```python
from build123d import *

# Parameters (mm, degrees)
F0_R     = 15.875
F1_DEPTH = 44.45
F2_SIZE  = 4.7625
F3_R     = 1.5875
F4_DEPTH = 17


with BuildPart() as f1:
    # F0 (on Front) → F1 (new body)
    with BuildSketch(Plane.XZ):
        Circle(F0_R)
    extrude(amount=F1_DEPTH)

    # F2
    f2_edges = [f1.edges().sort_by_distance(p)[0] for p in [
        (-15.875, -44.45, 0),
    ]]
    chamfer(f2_edges, length=F2_SIZE)

    # F3 (on face) → F4 (join)
    with BuildSketch(Plane.XZ.offset(44.45)):
        Circle(F3_R)
    extrude(amount=F4_DEPTH)


solid = f1.part
```
Model file for the job. Use its own axes, mm. A direction names the side the tool comes from. Coordinates: 2 decimals unless noted, no trailing zeros. Loops run counter-clockwise (first coordinate to the right, second up) from the corner with the lowest first, then second, coordinate; pieces in that order, holes last. Notation, with made-up numbers: (22.25, 45) - (47.25, 45) arc R21 cw to (47.25, 54) - close; hole circle Ø11 at (-4, 58). An arc over 180 degrees is marked (long way). Answer as a JSON object with one key per item and string values. Group by question number.
(1) Tool access for faces 1 (the face through (-0.34, -52.83, -1.55)), 2 (the face through (-3.441, -19.566, -15.497)): list every direction of +Z, -Z, +X, -X, +Y, -Y with a clear straight run to the whole face (end or side of a thin tool).
(2) Flat gauge pins, fed straight in: pin 1 (8 mm diameter, centred on x = 9.5, y = -34.5, fed in from -Z); pin 2 (3 mm diameter, centred on y = -20, z = 12.5, fed in from +X); pin 3 (12 mm diameter, centred on x = 10.5, y = -7, fed in from -Z). Where does each tip first touch, or does it go through?
(3) Cut at C-C (y = -35). Give the cut face in (x, z) (3 decimals), then the cut area to 3 significant figures.
(4) Cut at D-D (y = -48.5). Give the cut face in (x, z) (1 decimal).
(5) Probe line 1 along Y through (x, z) = (-6, -3.5); line 2 along X through (y, z) = (-21, 13); line 3 along Y through (x, z) = (-10, 8). List the from-to ranges inside material, lowest first.
Geometry says:
{
 "1": {"face 1": "-Y", "face 2": "+Y, -Y"},
 "2": {"pin 1": "stops at z = -14.89", "pin 2": "stops at x = 11.45", "pin 3": "stops at z = -15.22"},
 "3": {"outline": "circle Ø31.75 at (0, 0)", "area": "792 mm^2"},
 "4": {"outline": "circle Ø3.2 at (0, 0)"},
 "5": {"line 1": "y = -44.45 to 0", "line 2": "x = -9.11 to 9.11", "line 3": "y = -42.76 to 0"}
}
